For this review, take the finished solid that the model builds, in its own axes (mm). A direction names the side the tool comes from. Round coordinates to 2 decimals unless told otherwise and drop trailing zeros. Order: outer loops, then holes, each group sorted by start corner. A loop starts at its lowest first (then second) coordinate and runs counter-clockwise, first axis right, second up. Notation, with made-up numbers: M -24.75,48.25 L -1.75,48.25 A20 cw -1.75,78.25 Z; hole C 73,38.25 d6. An arc over 180 degrees is marked long. Answer in a Markdown table with one row per item. Add a question column.
```python
from build123d import *

# Parameters (mm, degrees)
F3_DEPTH  = 12.954
F1_R      = 13.7150037279
F0_R      = 27.1085366246
F4_DEPTH  = 25.4
F6_R      = 15.022792706
F7_W      = 16.4906103164
F7_H      = 6.7183971405
F8_DEPTH  = 56.134
F9_R      = 1.8396307345
F11_R     = 6.9234827164
F12_DEPTH = 40.894


with BuildPart() as f3:
    # F2 (on Top) → F3 (new body)
    with BuildSketch(Plane.XY):
        Polygon((-47.680426389, 27.2449441254), (-47.680426389, 0), (-47.925978899, -27.2676609457), (22.7930769324, -13.7622868642), (22.7930769324, 0), (22.7930769324, 14.2306741327), align=None)
    extrude(amount=F3_DEPTH)



with BuildPart() as f3b:
    # F1 (on Top) → F3, piece 2 (new body)
    with BuildSketch(Plane.XY):
        with Locations((23.2090074569, 0)):
            Circle(F1_R)
    extrude(amount=F3_DEPTH)


with BuildPart() as f3c:
    # F0 (on Top) → F3, piece 3 (new body)
    with BuildSketch(Plane.XY):
        with Locations((-47.0287799835, 0)):
            Circle(F0_R)
    extrude(amount=F3_DEPTH)


with BuildPart() as f3_1:
    add(f3.part)
    # F4 (add): a face of the model
    f4_faces = [f3c.part.faces().sort_by_distance(p)[0] for p in [
        (-47.0287799835, 0, 12.954),
    ]]

    add(f3b.part)  # F4 merges F3b

    add(f3c.part)  # F4 merges F3c
    extrude(f4_faces, amount=F4_DEPTH)

    # F6 (on offset) + F7 (on offset) → F8 (cut)
    with BuildSketch(Plane.XY.offset(48.514)):
        with Locations((-47.3341606557, 0)):
            Circle(F6_R)
    with BuildSketch(Plane.XY.offset(48.514)):
        with Locations((-31.1489319429, 0)):
            Rectangle(F7_W, F7_H)
    extrude(amount=-F8_DEPTH, mode=Mode.SUBTRACT)

    # F9
    f9_edges = [f3_1.edges().sort_by_distance(p)[0] for p in [
        (-74.137317, 0, 38.354),
    ]]
    fillet(f9_edges, radius=F9_R)

    # F11 (on offset) → F12 (cut)
    with BuildSketch(Plane.XY.offset(16.002)):
        with Locations((22.5982461125, 0)):
            Circle(F11_R)
    extrude(amount=-F12_DEPTH, mode=Mode.SUBTRACT)


solid = f3_1.part
```
1. Consider section B-B on z = 25.5. Write out the cut boundary in (x, y), plus the area to 3 significant figures.
2. For faces 5 (the cylindrical face through (-74.11, 1.19, 22.06)), 6 (the flat face through (-22.904, 0, 19)), 7 (the flat face through (-7.51, -19.55, 6.39)), list the 3-axis set-ups (+Z, -Z, +X, -X, +Y, -Y) from which the entire face can be reached by the end or side of a thin tool; tool diameter is ignored.
3. Consider section A-A on y = 0. Write out the cut boundary in (x, z).
4. To check wall thickness, follow probe 1 along X at (y, z) = (0, 24); probe 2 along Z at (x, y) = (-20, 16); probe 3 along X at (y, z) = (-11, 31). State the ranges of each line that lie inside material, in increasing order. Write a range as [from, to].
5. Clearance check with flat-ended pins moving along their axes: pin 1 Ø6 at (x, z) = (-7.5, 10.5) entering from -Y; pin 2 Ø8 at (x, z) = (-28.5, 28) entering from +Y; pin 3 Ø1 at (x, z) = (-24, 34) entering from +Y. State where each tip first meets the part, or that it passes through.
6. The part is to be moulded in two halves that separate along Y. For faces 1 (the flat face through (-1, 0, 12.954)), 2 (the flat face through (-6.896, 19.713, 6.386)), 3 (the cylindrical face through (36.92, -0.31, 6.39)), 4 (the flat face through (-28, -3.359, 19)), say which applies: pulls with the +Y half, pulls with the -Y half, needs draft (parallel to the pull), parting line crosses it, or undercut.
7. Consider section C-C on x = 4. Write out the cut boundary in (y, z), plus the area to 3 significant figures.
Solved:
| question | item | result |
|---|---|---|
| 1 | outline | C -47.03,0 d54.22; hole M -32.69,-3.36 L -22.9,-3.36 L -22.9,3.36 L -32.69,3.36 A15.02 ccw long Z |
| 1 | area | 1,540 mm^2 |
| 2 | face 5 | +Z |
| 2 | face 6 | +Z, -Z |
| 2 | face 7 | +Z, -Z, +X, -Y |
| 3 | outline | M -74.14,0 L -62.36,0 L -62.36,38.35 L -72.3,38.35 A1.84 ccw -74.14,36.51 Z; M -22.9,0 L 15.67,0 L 15.67,12.95 L -19.92,12.95 L -19.92,36.51 A1.84 ccw -21.76,38.35 L -22.9,38.35 Z; M 29.52,0 L 36.92,0 L 36.92,12.95 L 29.52,12.95 Z |
| 4 | probe 1 | x = [-74.14, -62.36], [-22.9, -19.92] |
| 4 | probe 2 | z = [0, 12.95] |
| 4 | probe 3 | x = [-71.81, -57.57], [-37.1, -22.25] |
| 5 | pin 1 | stops at y = -20.12 |
| 5 | pin 2 | stops at y = 22.89 |
| 5 | pin 3 | stops at y = 15.08 |
| 6 | face 1 | needs draft |
| 6 | face 2 | pulls with the +Y half |
| 6 | face 3 | parting line crosses it |
| 6 | face 4 | undercut |
| 7 | outline | M -17.35,0 L 17.7,0 L 17.7,12.95 L -17.35,12.95 Z |
| 7 | area | 454 mm^2 |
